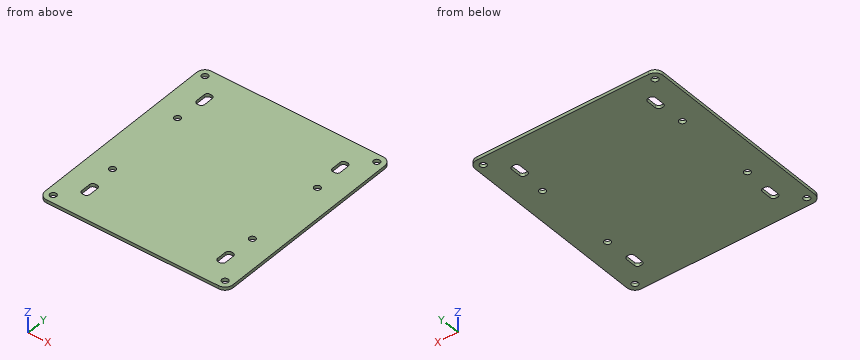
from build123d import *

# Parameters (mm, degrees)
SKETCH1_R           = 2
BOSS_EXTRUDE1_DEPTH = 2
CUT_EXTRUDE1_DEPTH  = 3


with BuildPart() as part:
    # Sketch1 → Boss-Extrude1 (new body)
    with BuildSketch(Plane.XY):
        with BuildLine():
            Line((69, -42.5), (176.5, -42.5))
            ThreePointArc((176.5, -42.5), (180.035533906, -43.964466094), (181.5, -47.5))
            Line((181.5, -47.5), (181.5, -166.5))
            ThreePointArc((181.5, -166.5), (180.035533906, -170.035533906), (176.5, -171.5))
            Line((176.5, -171.5), (69, -171.5))
            ThreePointArc((69, -171.5), (65.464466094, -170.035533906), (64, -166.5))
            Line((64, -166.5), (64, -47.5))
            ThreePointArc((64, -47.5), (65.464466094, -43.964466094), (69, -42.5))
        make_face()
        with Locations((166.5, -81.5)):
            Circle(SKETCH1_R, mode=Mode.SUBTRACT)
        with Locations((166.5, -132.5)):
            Circle(SKETCH1_R, mode=Mode.SUBTRACT)
        with Locations((79, -132.5)):
            Circle(SKETCH1_R, mode=Mode.SUBTRACT)
        with Locations((79, -81.5)):
            Circle(SKETCH1_R, mode=Mode.SUBTRACT)
        with Locations((69, -166.5)):
            Circle(SKETCH1_R, mode=Mode.SUBTRACT)
        with Locations((176.5, -166.5)):
            Circle(SKETCH1_R, mode=Mode.SUBTRACT)
        with Locations((176.5, -47.5)):
            Circle(SKETCH1_R, mode=Mode.SUBTRACT)
        with Locations((69, -47.5)):
            Circle(SKETCH1_R, mode=Mode.SUBTRACT)
    extrude(amount=BOSS_EXTRUDE1_DEPTH)

    # Sketch2 → Cut-Extrude1 (cut)
    with BuildSketch(Plane.XY.offset(2)):
        with BuildLine():
            Line((79.75, -57), (80.75, -57))
            ThreePointArc((80.75, -57), (82.164213562, -57.585786438), (82.75, -59))
            Line((82.75, -59), (82.75, -65))
            ThreePointArc((82.75, -65), (82.164213562, -66.414213562), (80.75, -67))
            Line((80.75, -67), (79.75, -67))
            ThreePointArc((79.75, -67), (78.335786438, -66.414213562), (77.75, -65))
            Line((77.75, -65), (77.75, -59))
            ThreePointArc((77.75, -59), (78.335786438, -57.585786438), (79.75, -57))
        make_face()
        with BuildLine():
            Line((162.75, -59), (162.75, -65))
            ThreePointArc((162.75, -65), (163.335786438, -66.414213562), (164.75, -67))
            Line((164.75, -67), (165.75, -67))
            ThreePointArc((165.75, -67), (167.164213562, -66.414213562), (167.75, -65))
            Line((167.75, -65), (167.75, -59))
            ThreePointArc((167.75, -59), (167.164213562, -57.585786438), (165.75, -57))
            Line((165.75, -57), (164.75, -57))
            ThreePointArc((164.75, -57), (163.335786438, -57.585786438), (162.75, -59))
        make_face()
        with BuildLine():
            Line((165.75, -157), (164.75, -157))
            ThreePointArc((164.75, -157), (163.335786438, -156.414213562), (162.75, -155))
            Line((162.75, -155), (162.75, -149))
            ThreePointArc((162.75, -149), (163.335786438, -147.585786438), (164.75, -147))
            Line((164.75, -147), (165.75, -147))
            ThreePointArc((165.75, -147), (167.164213562, -147.585786438), (167.75, -149))
            Line((167.75, -149), (167.75, -155))
            ThreePointArc((167.75, -155), (167.164213562, -156.414213562), (165.75, -157))
        make_face()
        with BuildLine():
            Line((82.75, -155), (82.75, -149))
            ThreePointArc((82.75, -149), (82.164213562, -147.585786438), (80.75, -147))
            Line((80.75, -147), (79.75, -147))
            ThreePointArc((79.75, -147), (78.335786438, -147.585786438), (77.75, -149))
            Line((77.75, -149), (77.75, -155))
            ThreePointArc((77.75, -155), (78.335786438, -156.414213562), (79.75, -157))
            Line((79.75, -157), (80.75, -157))
            ThreePointArc((80.75, -157), (82.164213562, -156.414213562), (82.75, -155))
        make_face()
    extrude(amount=-CUT_EXTRUDE1_DEPTH, mode=Mode.SUBTRACT)


solid = part.part
CAD build for the part. Positions are in the model's coordinates, mm. Round coordinates to 2 decimals unless told otherwise and drop trailing zeros. Write each loop counter-clockwise with the first axis right and the second up, starting at its lowest first coordinate (ties: lowest second). Pieces come first, ordered by that corner, then holes. Notation, with made-up numbers: (53, 9.25) -> (91, 9.25) arc R18 ccw to (91, 28.25) -> close; hole circle Ø2 at (47, 85). An arc over 180 degrees is marked (long way). Answer as a JSON object with one key per item and string values.
(1) Band-saw the part on A-A, the plane y = -132.5. List the corners of the cut face in (x, z), then the cut area to 3 significant figures.
Reported:
{"outline": "(64, 0) -> (77, 0) -> (77, 2) -> (64, 2) -> close; (81, 0) -> (164.5, 0) -> (164.5, 2) -> (81, 2) -> close; (168.5, 0) -> (181.5, 0) -> (181.5, 2) -> (168.5, 2) -> close", "area": "219 mm^2"}
(2) Band-saw the part on B-B, the plane z = 1.25. Count the separate pieces of the cut face and the enclosed holes in it, then the cut area to 3 significant figures.
Reported:
{"separate pieces": "1", "enclosed holes": "12", "area": "14,800 mm^2"}
(3) Probe probe 1 along Y at (x, z) = (176.5, 0.5); probe 2 along X at (y, z) = (-166.5, 0.5); probe 3 along X at (y, z) = (-80.5, 1.6). List the from-to ranges inside material, lowest first. Write a range as [from, to].
Reported:
{"probe 1": "y = [-171.5, -168.5], [-164.5, -49.5], [-45.5, -42.5]", "probe 2": "x = [64, 67], [71, 174.5], [178.5, 181.5]", "probe 3": "x = [64, 77.27], [80.73, 164.77], [168.23, 181.5]"}
(4) Pin check, flat tips, straight feed: P1, Ø3, axis at x = 79, y = -132.5, coming from the -Z side; P2, Ø4.5, axis at x = 79, y = -81.5, coming from the -Z side. Stop position of each tip, or through.
Reported:
{"P1": "passes through", "P2": "stops at z = 0"}
